Verification items for the finished model (mm, model axes). A direction names the side the tool comes from. Coordinates: 2 decimals unless noted, no trailing zeros. Write each loop counter-clockwise with the first axis right and the second up, starting at its lowest first coordinate (ties: lowest second). Pieces come first, ordered by that corner, then holes. Notation, with made-up numbers: (-29.75, 46.25) -> (-2.75, 46.25) arc R21 cw to (-2.75, 84.25) -> close; hole circle Ø8 at (-33.5, 40.25). An arc over 180 degrees is marked (long way). Use a Markdown table: item, result. Add a question column.
from build123d import *

# Parameters (mm, degrees)
BOSS_EXTRUDE1_DEPTH = 25.4
SKETCH2_R           = 4.7625
CUT_EXTRUDE1_DEPTH  = 25.4
SKETCH3_R           = 4.7625
CUT_EXTRUDE2_DEPTH  = 4.175


with BuildPart() as part:
    # Sketch1 → Boss-Extrude1 (new body)
    with BuildSketch(Plane(origin=(0, 0, 0), x_dir=(0, 0, -1), z_dir=(1, 0, 0))):
        Polygon((0, 0), (-25.4, 0), (-25.4, 3.175), (-3.175, 3.175), (-3.175, 25.4), (0, 25.4), align=None)
    extrude(amount=BOSS_EXTRUDE1_DEPTH)

    # Sketch2 → Cut-Extrude1 (cut)
    with BuildSketch(Plane(origin=(0, 3.175, 0), x_dir=(1, 0, 0), z_dir=(0, 1, 0))):
        with Locations((12.7, -12.7)):
            Circle(SKETCH2_R)
    extrude(amount=-CUT_EXTRUDE1_DEPTH, mode=Mode.SUBTRACT)

    # Sketch3 → Cut-Extrude2 (cut, through all)
    with BuildSketch(Plane.XY.offset(3.175)):
        with Locations((12.7, 12.7)):
            Circle(SKETCH3_R)
    extrude(amount=-CUT_EXTRUDE2_DEPTH, mode=Mode.SUBTRACT)


solid = part.part
1) Cross-section at A-A on y = 12.7. Record the boundary of the cut face in (x, z) (1 decimal).
2) Cross-section at D-D on z = 2. Record the boundary of the cut face in (x, y) (1 decimal), then the cut area to 3 significant figures.
3) Release check for a two-part mould opening along Y. For faces 3 (the face through (13, 25.4, 2)), 4 (the face through (13, 0, 18)), 5 (the face through (7.942, 12.909, 1.61)), 6 (the face through (7.942, 1.61, 12.491)) record: released by +Y, released by -Y, zero draft, split by the parting line, or undercut.
4) Gauge pin test, flat ends, axial feed: pin 1 (1 mm diameter, centred on x = 20.5, z = 19.5, fed in from +Y) (3 decimals); pin 2 (2 mm diameter, centred on x = 10.5, y = 4.5, fed in from +Z) (3 decimals). Record the tip position at first contact, or that the pin passes through.
5) Cross-section at C-C on x = 9. Record the boundary of the cut face in (y, z) (3 decimals), then the cut area to 3 significant figures.
6) Set-up check for faces 1 (the face through (10, 17, 3.175)), 2 (the face through (13, 7, 0)): record each of +Z, -Z, +X, -X, +Y, -Y from which the full face is reachable in a straight line by a thin tool's end or side.
7) Thickness scan on L1, parallel to Y at x = 12.7, z = 1.3; L2, parallel to Y at x = 1.25, z = 5.25 (3 decimals). Record the ranges inside material, lowest first.
Returned:
| question | item | result |
|---|---|---|
| 1 | outline | (0, 0) -> (7.9, 0) -> (7.9, 3.2) -> (0, 3.2) -> close; (17.5, 0) -> (25.4, 0) -> (25.4, 3.2) -> (17.5, 3.2) -> close |
| 2 | outline | (0, 0) -> (25.4, 0) -> (25.4, 25.4) -> (0, 25.4) -> close; hole circle Ø9.5 at (12.7, 12.7) |
| 2 | area | 574 mm² |
| 3 | face 3 | released by +Y |
| 3 | face 4 | released by -Y |
| 3 | face 5 | undercut |
| 3 | face 6 | zero draft |
| 4 | pin 1 | stops at y = 3.175 |
| 4 | pin 2 | stops at z = 3.175 |
| 5 | outline | (0, 0) -> (9.701, 0) -> (9.701, 3.175) -> (3.175, 3.175) -> (3.175, 9.701) -> (0, 9.701) -> close; (0, 15.699) -> (3.175, 15.699) -> (3.175, 25.4) -> (0, 25.4) -> close; (15.699, 0) -> (25.4, 0) -> (25.4, 3.175) -> (15.699, 3.175) -> close |
| 5 | area | 113 mm² |
| 6 | face 1 | +Z, +X, -X, +Y |
| 6 | face 2 | -Z, +X, -X, +Y, -Y |
| 7 | L1 | y = 0 to 7.94, 17.46 to 25.4 |
| 7 | L2 | y = 0 to 3.175 |
